For this review, use the dimensioned drawing (mm, ordinates from the lowest corner) and the shaded views. Give positions to 0.01 mm unless a question says otherwise; leave off trailing zeros. Loops run counter-clockwise (first coordinate to the right, second up) from the corner with the lowest first, then second, coordinate; pieces in that order, holes last. Notation, with made-up numbers: (53, 38) - (94, 38) arc R12 cw to (94, 53) - close; hole circle Ø7 at (42.5, 60.5). An arc over 180 degrees is marked (long way). Put each result on its own line as item: value.
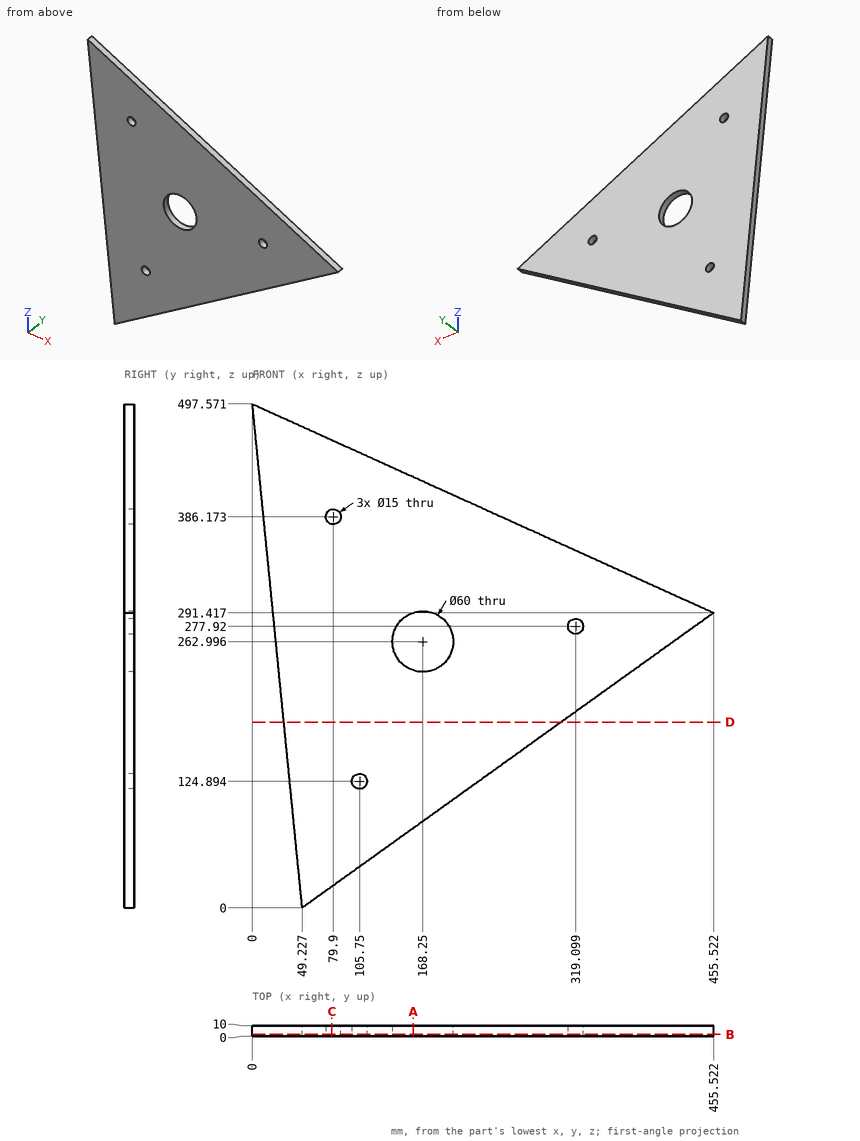
1) Wall thickness on line 1 (X direction, y = 6, z = 388) (1 decimal); line 2 (Z direction, x = 149.5, y = 5.75) (1 decimal); line 3 (X direction, y = 1.5, z = 273) (1 decimal): over which ranges is each line inside the solid? List them lowest first.
Geometry check:
line 1: x = 10.8 to 72.6, 87.2 to 242.1
line 2: z = 71.9 to 239.6, 286.4 to 429.9
line 3: x = 22.2 to 140, 196.5 to 313.4, 324.8 to 429.8
2) Take a section at C-C on x = 78.5. State the section outline as (y, z) points (1 decimal).
Geometry check:
outline: (0, 21) - (10, 21) - (10, 378.8) - (0, 378.8) - close; (0, 393.5) - (10, 393.5) - (10, 462) - (0, 462) - close
3) Take a section at D-D on z = 183.5. State the section outline as (x, y) points, and give its area (3 significant figures).
Geometry check:
outline: (31.07, 0) - (305.06, 0) - (305.06, 10) - (31.07, 10) - close
area: 2,740 mm²
4) Insertion check: pin 1 Ø6 at (x, y) = (269, 3.5) entering from +Z; pin 2 Ø2 at (x, y) = (346.5, 2) entering from +Z; pin 3 Ø24 at (x, z) = (79.9, 386.17) entering from -Y; pin 4 Ø5 at (y, z) = (2, 282) entering from +X. Each pin has a flat end and moves straight along its axis. Give the tip position at first contact, or say it passes through.
Geometry check:
pin 1: stops at z = 377.19
pin 2: stops at z = 341.21
pin 3: stops at y = 0
pin 4: stops at x = 445.88
5) Take a section at B-B on y = 1.5. State how many separate pieces and enclosed holes the cut face has, and give its area (3 significant figures).
Geometry check:
separate pieces: 1
enclosed holes: 4
area: 105,000 mm²
6) Take a section at A-A on x = 159. State the section outline as (y, z) points (1 decimal), and give its area (3 significant figures).
Geometry check:
outline: (0, 78.7) - (10, 78.7) - (10, 234.5) - (0, 234.5) - close; (0, 291.5) - (10, 291.5) - (10, 425.6) - (0, 425.6) - close
area: 2,900 mm²
